from build123d import *
from build123d.topology import SkipClean

# Parameters (mm, degrees)
EXTRUDE_1_DEPTH     = 0.5
EXTRUDE_2_DEPTH     = 6.4
EXTRUDE_3_DEPTH     = 0.5
EXTRUDE_START       = -7.4
EXTRUDE_6_DEPTH     = 7.4
SKETCH_16_W         = 0.8
SKETCH_16_H         = 12
EXTRUDE_10_DEPTH    = 6.4
EXTRUDE_11_DEPTH    = 0.5
CUT_EXTRUDE_START   = -3
CUT_EXTRUDE_1_DEPTH = 3
CUT_EXTRUDE_2_DEPTH = 3


# Read off the part's stored shape, not the designer's step: 凸台-拉伸2
with BuildPart() as part:
    # 草图1 → 凸台-拉伸1 (new body)
    with BuildSketch(Plane(origin=(0, 0, 0), x_dir=(1, 0, 0), z_dir=(0, 1, 0))):
        with BuildLine():
            Line((11.456239028, 1.002291042), (10.46004433, 0.915135299))
            ThreePointArc((10.46004433, 0.915135299), (-10.5, 0), (10.46004433, -0.915135299))
            Line((10.46004433, -0.915135299), (11.456239028, -1.002291042))
            ThreePointArc((11.456239028, -1.002291042), (5.310109052, -10.200624582), (-5.75, -9.959292144))
            ThreePointArc((-5.75, -9.959292144), (-8.028256991, -8.233898814), (-9.810708435, -6))
            Line((-9.810708435, -6), (-13.5, -6))
            Line((-13.5, -6), (-13.5, 0))
            Line((-13.5, 0), (-13.5, 6))
            Line((-13.5, 6), (-9.810708435, 6))
            ThreePointArc((-9.810708435, 6), (-8.028256991, 8.233898814), (-5.75, 9.959292144))
            ThreePointArc((-5.75, 9.959292144), (5.310109052, 10.200624582), (11.456239028, 1.002291042))
        make_face()
    extrude(amount=EXTRUDE_1_DEPTH)

    # 凸台-拉伸2 outline → 凸台-拉伸2 (add)
    with BuildSketch(Plane(origin=(0, 0.5, 0), x_dir=(1, 0, 0), z_dir=(0, 1, 0))):
        with BuildLine():
            ThreePointArc((11.456239028, 1.002291042), (-11.5, 0), (11.456239028, -1.002291042))
            Line((11.456239028, -1.002291042), (10.46004433, -0.915135299))
            ThreePointArc((10.46004433, -0.915135299), (-10.5, 0), (10.46004433, 0.915135299))
            Line((10.46004433, 0.915135299), (11.456239028, 1.002291042))
        make_face()
    extrude(amount=EXTRUDE_2_DEPTH)

    # 草图11 → 凸台-拉伸3 (add)
    with BuildSketch(Plane(origin=(0, 6.9, 0), x_dir=(1, 0, 0), z_dir=(0, 1, 0))):
        with BuildLine():
            Line((10.46004433, 0.915135299), (11.456239028, 1.002291042))
            ThreePointArc((11.456239028, 1.002291042), (-11.5, 0), (11.456239028, -1.002291042))
            Line((11.456239028, -1.002291042), (10.46004433, -0.915135299))
            ThreePointArc((10.46004433, -0.915135299), (-10.5, 0), (10.46004433, 0.915135299))
        make_face()
    extrude(amount=EXTRUDE_3_DEPTH)

    # 草图14 → 凸台-拉伸6 (add)
    with SkipClean():  # the faces are left unmerged after this step: merging them gives an invalid solid
        with BuildSketch(Plane(origin=(0, 7.4, 0), x_dir=(1, 0, 0), z_dir=(0, 1, 0)).offset(EXTRUDE_START)):
            with BuildLine():
                Line((10.46004433, 0.915135299), (11.456239028, 1.002291042))
                ThreePointArc((11.456239028, 1.002291042), (11.5, 0), (11.456239028, -1.002291042))
                Line((11.456239028, -1.002291042), (10.46004433, -0.915135299))
                ThreePointArc((10.46004433, -0.915135299), (10.5, 0), (10.46004433, 0.915135299))
            make_face()
        extrude(amount=EXTRUDE_6_DEPTH)
    add(part.part.scale(1), mode=Mode.REPLACE)  # the faces are merged on a copy

    # 草图16 → 凸台-拉伸10 (add)
    with BuildSketch(Plane(origin=(0, 0.5, 0), x_dir=(1, 0, 0), z_dir=(0, 1, 0))):
        with Locations((-13.1, 0)):
            Rectangle(SKETCH_16_W, SKETCH_16_H)
    extrude(amount=EXTRUDE_10_DEPTH)

    # 草图17 → 凸台-拉伸11 (add)
    with BuildSketch(Plane(origin=(0, 6.9, 0), x_dir=(1, 0, 0), z_dir=(0, 1, 0))):
        with BuildLine():
            Line((-13.5, 6), (-9.810708435, 6))
            ThreePointArc((-9.810708435, 6), (-11.5, 0), (-9.810708435, -6))
            Line((-9.810708435, -6), (-13.5, -6))
            Line((-13.5, -6), (-13.5, 6))
        make_face()
    extrude(amount=EXTRUDE_11_DEPTH)

    # 草图18 → 切除-拉伸1 (cut)
    with BuildSketch(Plane(origin=(0, 7.4, 0), x_dir=(1, 0, 0), z_dir=(0, 1, 0)).offset(CUT_EXTRUDE_START)):
        with BuildLine():
            Line((-9.810708435, 6), (-8.957603354, 5.47826087))
            ThreePointArc((-8.957603354, 5.47826087), (10.5, 0), (-8.957603354, -5.47826087))
            Line((-8.957603354, -5.47826087), (-9.810708435, -6))
            ThreePointArc((-9.810708435, -6), (11.5, 0), (-9.810708435, 6))
        make_face()
    extrude(amount=CUT_EXTRUDE_1_DEPTH, mode=Mode.SUBTRACT)

    # 草图19 → 切除-拉伸2 (cut)
    with BuildSketch(Plane(origin=(0, 0, 0), x_dir=(-1, 0, 0), z_dir=(0, -1, 0))):
        with BuildLine():
            Line((9.810708435, 6), (8.957603354, 5.47826087))
            ThreePointArc((8.957603354, 5.47826087), (-10.5, 0), (8.957603354, -5.47826087))
            Line((8.957603354, -5.47826087), (9.810708435, -6))
            ThreePointArc((9.810708435, -6), (-11.5, 0), (9.810708435, 6))
        make_face()
    extrude(amount=-CUT_EXTRUDE_2_DEPTH, mode=Mode.SUBTRACT)


solid = part.part
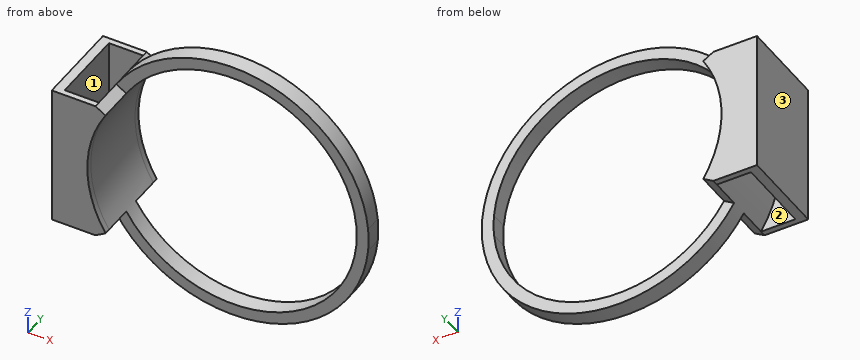
Geometry check sheet. Reference: the model listing, model coordinates, mm. Face numbers are marked on the shaded views. A direction names the side the tool comes from. Give positions to 0.01 mm unless a question says otherwise; leave off trailing zeros. Write each loop counter-clockwise with the first axis right and the second up, starting at its lowest first coordinate (ties: lowest second). Pieces come first, ordered by that corner, then holes. Notation, with made-up numbers: M -23.5,42 L 16.5,42 A10 ccw 16.5,58 Z; hole C -4.5,11 d3. An arc over 180 degrees is marked long. Answer as CSV lines item,"result". Start each with the question number.
Q1. Material ranges on L1, parallel to Z at x = 0, y = 3.5; L2, parallel to X at y = 5, z = 0; L3, parallel to X at y = 3.75, z = -4.25, recorded low to high.
Q2. Section check B-B, the plane x = 0. Record the cut outline in (y, z).
Q3. Section check A-A, the plane y = 3.5. Record the cut outline in (x, z).
Q4. Section check C-C, the plane z = 0. Record the cut outline in (x, y).
Q5. Go/stop test with flat-tipped pins: pin 1 (3 mm diameter, centred on x = -11.5, y = 4.5, fed in from -Z); pin 2 (6 mm diameter, centred on x = 8.5, z = -7.5, fed in from +Y); pin 3 (1.5 mm diameter, centred on x = 5, z = -7.5, fed in from +Y). Record where each tip stops, or that it passes through.
Q6. Tool access check on the marked faces 1, 2 and 3. Record the directions out of +Z, -Z, +X, -X, +Y, -Y that give a thin tool (end or side, any length) a straight path to the whole face; none if there is none.
Q7. Section check D-D, the plane y = 1. Record the cut outline in (x, z).
Geometry says:
1,L1,"-11.5 to -10.5, 10.5 to 11.5"
1,L2,"-13.5 to -12.7, -11.5 to -10.5"
1,L3,"-13.5 to -12.7, -10.69 to -9.6, 9.6 to 10.69"
2,outline,"M 3,-11.5 L 4.4,-11.5 L 4.4,-10.5 L 3,-10.5 Z; M 3,10.5 L 4.4,10.5 L 4.4,11.5 L 3,11.5 Z"
3,outline,"M -13.5,-6 L -12.7,-6 L -12.7,6 L -13.5,6 Z; C 0,0 d23; hole C 0,0 d21"
4,outline,"M -13.5,0 L -10.5,0 L -10.5,7.4 L -13.5,7.4 Z; M 10.5,3 L 11.5,3 L 11.5,4.4 L 10.5,4.4 Z; hole M -12.7,0.5 L -11.5,0.5 L -11.5,6.9 L -12.7,6.9 Z"
5,pin 1,"z = -6"
5,pin 2,"y = 4.4"
5,pin 3,"through"
6,face 1,"+Z, -Z"
6,face 2,"none"
6,face 3,"+Z, -Z, -X, +Y, -Y"
7,outline,"M -13.5,-6 L -12.7,-6 L -12.7,6 L -13.5,6 Z; M -9.81,-6 L -8.96,-5.48 A10.5 cw -8.96,5.48 L -9.81,6 A11.5 ccw Z"
